Study the drawing (mm; zero at the part's minimum x, y, z) and answer. A direction names the side the tool comes from. Coordinates: 2 decimals unless noted, no trailing zeros. Order: outer loops, then holes, each group sorted by start corner. A loop starts at its lowest first (then second) coordinate and runs counter-clockwise, first axis right, second up.
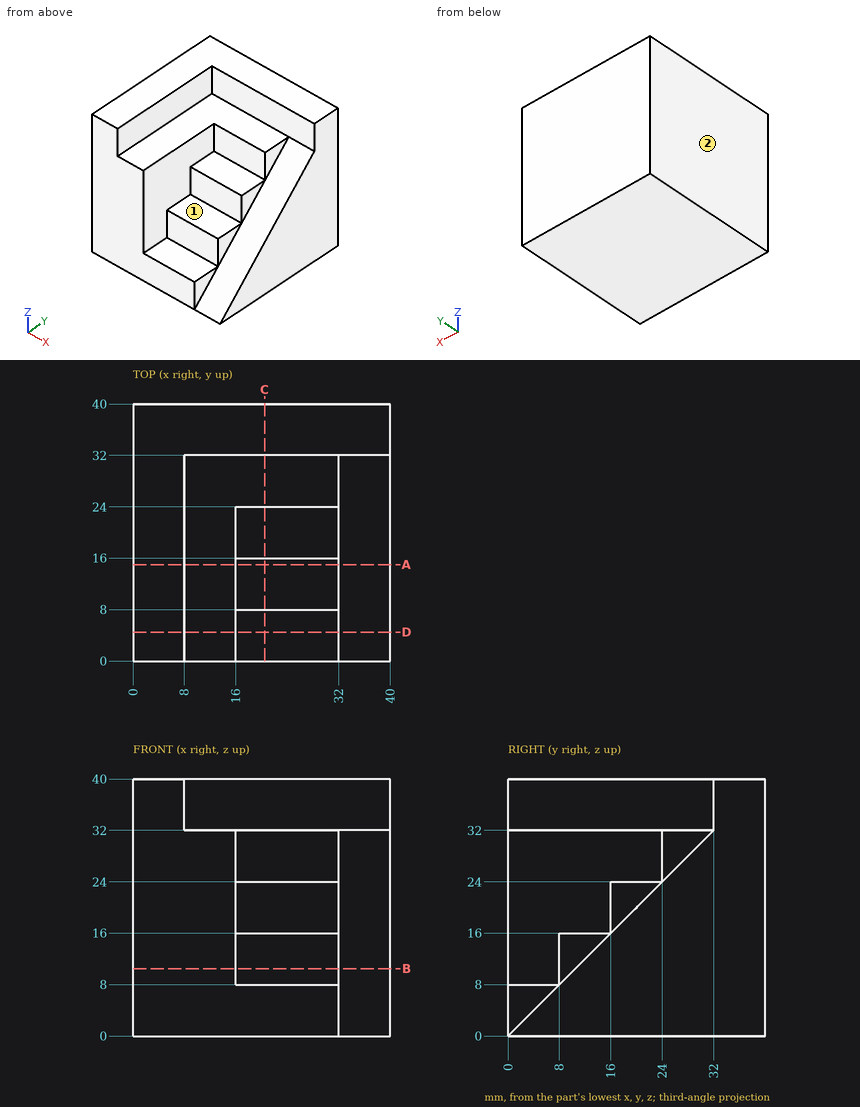
(1) Find section A-A on y = 15. Determine the outline of the cut face in (x, z), then the cut area to 3 significant figures.
(2) Find section D-D on y = 4.5. Determine the outline of the cut face in (x, z).
(3) Given pin 1 Ø19 at (y, z) = (12.5, 18.5) entering from +X; pin 2 Ø19 at (x, y) = (25, 22) entering from +Z; pin 3 Ø6 at (y, z) = (8, 22) entering from +X; pin 4 Ø6.5 at (y, z) = (13, 36.5) entering from +X, each flat-ended and moving along its own axis, determine where each tip first touches the part or whether it passes through.
(4) Find section B-B on z = 10.5. Determine the outline of the cut face in (x, y).
(5) Find the intervals of material crossed by probe 1 along X at (y, z) = (4, 14); probe 2 along Y at (x, z) = (16, 34); probe 3 along Y at (x, z) = (20, 30), in increasing order.
(6) Find section C-C on x = 20.5. Determine the outline of the cut face in (y, z), then the cut area to 3 significant figures.
(7) A tool of negligible diameter and unlimited length cuts with its end or side. For the marked faces 1 and 2, from which of +Z, -Z, +X, -X, +Y, -Y can it reach the whole face along a straight path? Write none if from no direction.
Resolved:
1. outline: (0, 0) - (40, 0) - (40, 15) - (32, 15) - (32, 16) - (16, 16) - (16, 32) - (8, 32) - (8, 40) - (0, 40) - close
1. area: 952 mm2
2. outline: (0, 0) - (40, 0) - (40, 4.5) - (32, 4.5) - (32, 8) - (16, 8) - (16, 32) - (8, 32) - (8, 40) - (0, 40) - close
3. pin 1: stops at x = 40
3. pin 2: stops at z = 32
3. pin 3: stops at x = 16
3. pin 4: stops at x = 8
4. outline: (0, 0) - (16, 0) - (16, 8) - (32, 8) - (32, 10.5) - (40, 10.5) - (40, 40) - (0, 40) - close
5. probe 1: x = 0 to 16
5. probe 2: y = 32 to 40
5. probe 3: y = 24 to 40
6. outline: (0, 0) - (40, 0) - (40, 40) - (32, 40) - (32, 32) - (24, 32) - (24, 24) - (16, 24) - (16, 16) - (8, 16) - (8, 8) - (0, 8) - close
6. area: 960 mm2
7. face 1: +Z, +X, -Y
7. face 2: +Z, -Z, -X, +Y, -Y
